The listing builds one solid part. Answer for the finished solid, in the listing's coordinates (mm). Coordinates: 2 decimals unless noted, no trailing zeros. Answer as CSV lines item,"result". Start each with the question number.
```python
from build123d import *

# Parameters (mm, degrees)
EXTRUSION1_DEPTH       = 350
SKETCH_2_R             = 3
SKETCH_2_R_2           = 1.75
CUT_EXTRUDE_1_DEPTH    = 4.5
SKETCH_2_2_R           = 1.75
CUT_EXTRUDE_2_DEPTH    = 351.142828
PATTERN_LINEAR_1_COUNT = 14
PATTERN_LINEAR_1_PITCH = 25


with BuildPart() as part:
    # Sketch 1 → Extrusion1 (new body)
    with BuildSketch(Plane.XY):
        with BuildLine():
            Line((-6, 3.7), (-5.7, 4))
            Line((-5.7, 4), (5.7, 4))
            Line((5.7, 4), (6, 3.7))
            Line((6, 3.7), (6, 2.451013544))
            ThreePointArc((6, 2.451013544), (5.597935912, 2.202976267), (5.354599002, 1.798050138))
            Line((5.354599002, 1.798050138), (4.643514056, 1.798050138))
            Line((4.643514056, 1.798050138), (4.643514056, 1.201949862))
            Line((4.643514056, 1.201949862), (5.354599002, 1.201949862))
            ThreePointArc((5.354599002, 1.201949862), (5.597935912, 0.797023733), (6, 0.548986456))
            Line((6, 0.548986456), (6, -3.7))
            Line((6, -3.7), (5.7, -4))
            Line((5.7, -4), (-5.7, -4))
            Line((-5.7, -4), (-6, -3.7))
            Line((-6, -3.7), (-6, 0.548986456))
            ThreePointArc((-6, 0.548986456), (-5.597935912, 0.797023733), (-5.354599002, 1.201949862))
            Line((-5.354599002, 1.201949862), (-4.643514056, 1.201949862))
            Line((-4.643514056, 1.201949862), (-4.643514056, 1.798050138))
            Line((-4.643514056, 1.798050138), (-5.354599002, 1.798050138))
            ThreePointArc((-5.354599002, 1.798050138), (-5.597935912, 2.202976267), (-6, 2.451013544))
            Line((-6, 2.451013544), (-6, 3.7))
        make_face()
    extrude(amount=EXTRUSION1_DEPTH)

    # Sketch 2 → Cut-Extrude 1 (cut)
    with BuildSketch(Plane(origin=(0, 4, 0), x_dir=(1, 0, 0), z_dir=(0, 1, 0))):
        with Locations(Location((0, -12.5, 0), (0, 0, 270))):
            Circle(SKETCH_2_R)
        with Locations(Location((0, -12.5, 0), (0, 0, 270))):
            Circle(SKETCH_2_R_2, mode=Mode.SUBTRACT)
    cut_extrude_1 = extrude(amount=-CUT_EXTRUDE_1_DEPTH, mode=Mode.SUBTRACT)

    # Sketch 2_2 → Cut-Extrude 2 (cut, through all)
    with BuildSketch(Plane(origin=(0, 4, 0), x_dir=(1, 0, 0), z_dir=(0, 1, 0))):
        with Locations(Location((0, -12.5, 0), (0, 0, 270))):
            Circle(SKETCH_2_2_R)
    cut_extrude_2 = extrude(amount=-CUT_EXTRUDE_2_DEPTH, mode=Mode.SUBTRACT)

    # Pattern Linear 1: Cut-Extrude 1, Cut-Extrude 2 ×14
    with Locations(*[(0, 0, i * PATTERN_LINEAR_1_PITCH) for i in range(1, PATTERN_LINEAR_1_COUNT)]):
        add(cut_extrude_1, mode=Mode.SUBTRACT)
        add(cut_extrude_2, mode=Mode.SUBTRACT)


solid = part.part
```
1) Find the intervals of material crossed by line 1 (X direction, y = -2.15, z = 62.5); line 2 (X direction, y = 1.45, z = 187.5); line 3 (X direction, y = 2.25, z = 41), in increasing order. Write a range as from..to.
2) For a pull along X with two mould halves and no side action, classify faces 1 (the face through (0, 4, 173)), 2 (the face through (-2, -0.5, 162)) as +X half, -X half, draft (parallel to the pull), parting line (faces both ways), or undercut.
3) Each of these flat-tipped pins is pushed along its axis until it touches: P1, Ø4, axis at x = 0, z = 287.5, coming from the +Y side; P2, Ø3, axis at x = 0, z = 87.5, coming from the +Y side; P3, Ø0.5, axis at y = 1.5, z = 162.5, coming from the -X side. Where does it stop, or does it pass through?
4) The part is cut by section A-A (y = -2). Count the separate pieces of the cut face and the enclosed holes in it, then the cut area to 3 significant figures.
Completed:
1,line 1,"-6..-1.75, 1.75..6"
1,line 2,"-4.64..-3, 3..4.64"
1,line 3,"-5.65..5.65"
2,face 1,"draft"
2,face 2,"undercut"
3,P1,"y = -0.5"
3,P2,"through"
3,P3,"x = -4.64"
4,separate pieces,"1"
4,enclosed holes,"14"
4,area,"4,070 mm²"
